Can you work these out from the model? Positions are in its coordinate system, mm. A direction names the side the tool comes from. Coordinates: 2 decimals unless noted, no trailing zeros. Loops run counter-clockwise (first coordinate to the right, second up) from the corner with the lowest first, then second, coordinate; pieces in that order, holes last. Notation, with made-up numbers: (40, -28.5) -> (77, -28.5) arc R23 ccw to (77, 9.5) -> close; hole circle Ø6 at (-19, 16.25). An arc over 180 degrees is marked (long way). Put each result on its own line as item: value. Start each with the question number.
Item 1: If we section it at C-C on z = 133: Please give me the cut outline in (x, y) (3 decimals), plus the area to 3 significant figures.
Item 2: For faces 5 (the flat face through (133, 36, -152.4)), 6 (the flat face through (114.3, 36, 134)), 7 (the flat face through (133, 36, 114.3)), 8 (the flat face through (134, 0, 134)), 9 (the flat face through (-114.3, 104, -134)), which set-ups out of +Z, -Z, +X, -X, +Y, -Y let a thin tool reach every point of the face, with its end or its side?
Item 3: We'd pull the mould along Z, two halves only. Please class faces 1 (the flat face through (-133, 36, 152.4)), 2 (the flat face through (2, 105, -152.4)), 3 (the flat face through (-152.4, 36, 134)), 4 (the flat face through (-152.4, 105, -2)): pulls with the +Z half, pulls with the -Z half, needs draft (parallel to the pull), parting line crosses it, or undercut.
Item 4: Will these pins go through, and if not, where does the flat tip stop? P1, Ø2, axis at x = -43.5, z = 49, coming from the -Y side; P2, Ø12, axis at x = 122.5, z = -44.5, coming from the +Y side; P3, Ø19, axis at y = 21, z = -125.5, coming from the +X side.
Item 5: If we section it at A-A on y = 56.5: Please give me the cut outline in (x, z).
Item 6: If we section it at B-B on y = 100: Please give me the cut outline in (x, z), plus the area to 3 significant figures.
Item 7: If we section it at D-D on x = 137: Please give me the cut outline in (y, z) (3 decimals), plus the area to 3 significant figures.
Item 8: Please list where these lines run through material, in increasing order: L1, parallel to X at y = 87, z = 33; L2, parallel to X at y = 69.5, z = -149.5. Write a range as from..to.
Autodesk Inventor part; units mm, degrees
ref_plane "YZ Plane" through (0, 0, 0) normal (1, 0, 0) x (0, 1, 0)
ref_plane "XZ Plane" through (0, 0, 0) normal (0, 1, 0) x (-1, 0, 0)
ref_plane "XY Plane" through (0, 0, 0) normal (0, 0, 1) x (1, 0, 0)
sketch "Sketch1" plane through (0, 0, 0) normal (0, 1, 0) x (-1, 0, 0)
  line L0 (-152.4, 152.4) -> (152.4, 152.4) construction
  line L1 (152.4, 152.4) -> (152.4, -152.4) construction
  line L2 (152.4, -152.4) -> (-152.4, -152.4) construction
  line L3 (-152.4, -152.4) -> (-152.4, 152.4) construction
  line L4 (-152.4, 152.4) -> (152.4, -152.4) construction
  line L5 (152.4, 152.4) -> (-152.4, -152.4) construction
  line L6 (152.4, -152.4) -> (114.3, -152.4)
  line L7 (114.3, -152.4) -> (114.3, -114.3)
  line L8 (114.3, -114.3) -> (152.4, -114.3)
  line L9 (152.4, -114.3) -> (152.4, -152.4)
  line L10 (152.4, 152.4) -> (152.4, 114.3)
  line L11 (152.4, 114.3) -> (114.3, 114.3)
  line L12 (114.3, 114.3) -> (114.3, 152.4)
  line L13 (114.3, 152.4) -> (152.4, 152.4)
  line L14 (-152.4, 152.4) -> (-114.3, 152.4)
  line L15 (-114.3, 152.4) -> (-114.3, 114.3)
  line L16 (-114.3, 114.3) -> (-152.4, 114.3)
  line L17 (-152.4, 114.3) -> (-152.4, 152.4)
  line L18 (-152.4, -152.4) -> (-152.4, -114.3)
  line L19 (-152.4, -114.3) -> (-114.3, -114.3)
  line L20 (-114.3, -114.3) -> (-114.3, -152.4)
  line L21 (-114.3, -152.4) -> (-152.4, -152.4)
  point P0 (0, 0)
  dimension "d0" = 304.8
  dimension "d1" = 304.8
  dimension "d2" = 38.1
  dimension "d5" = 360
extrude "Extrusion1" add sketch "Sketch1" along normal blind 127
sketch "Sketch2" plane through (0, 127, 0) normal (0, 1, 0) x (1, 0, 0)
  line L0 (-114.3, 152.4) -> (-152.4, 152.4)
  line L1 (-152.4, 152.4) -> (-152.4, 114.3)
  line L2 (-152.4, 114.3) -> (-114.3, 114.3)
  line L3 (-114.3, 114.3) -> (-114.3, 152.4)
  line L4 (152.4, 114.3) -> (152.4, 152.4)
  line L5 (152.4, 152.4) -> (114.3, 152.4)
  line L6 (114.3, 152.4) -> (114.3, 114.3)
  line L7 (114.3, 114.3) -> (152.4, 114.3)
  line L8 (114.3, -152.4) -> (152.4, -152.4)
  line L9 (152.4, -152.4) -> (152.4, -114.3)
  line L10 (152.4, -114.3) -> (114.3, -114.3)
  line L11 (114.3, -114.3) -> (114.3, -152.4)
  line L12 (-152.4, -114.3) -> (-152.4, -152.4)
  line L13 (-152.4, -152.4) -> (-114.3, -152.4)
  line L14 (-114.3, -152.4) -> (-114.3, -114.3)
  line L15 (-114.3, -114.3) -> (-152.4, -114.3)
  line L16 (0, 231.14) -> (0, -231.14)
  line L17 (231.14, 0) -> (-231.14, 0)
  line L18 (-152.4, 152.4) -> (-152.4, -152.4)
  line L19 (-152.4, -152.4) -> (152.4, -152.4)
  line L20 (152.4, -152.4) -> (152.4, 152.4)
  line L21 (152.4, 152.4) -> (-152.4, 152.4)
  line L22 (-165.1, 165.1) -> (-165.1, -165.1)
  line L23 (-165.1, -165.1) -> (165.1, -165.1)
  line L24 (165.1, -165.1) -> (165.1, 165.1)
  line L25 (165.1, 165.1) -> (-165.1, 165.1)
  point P0 (0, 0)
  dimension "d9" = 12.7
extrude "Extrusion2" add sketch "Sketch2" against normal blind 57.15 contours L0 L1 L18 L17 L22 L25 L16 L21 | L16 L25 L24 L17 L20 L4 L5 L21 | L18 L12 L13 L19 L16 L23 L22 L17 | L19 L8 L9 L20 L17 L24 L23 L16
sketch "Sketch3" plane through (0, 69.85, 0) normal (0, -1, 0) x (1, 0, 0)
  line L0 (-165.1, 165.1) -> (165.1, 165.1)
  line L1 (-165.1, -165.1) -> (-165.1, 165.1)
  line L2 (-165.1, 165.1) -> (165.1, 165.1)
  line L3 (165.1, 165.1) -> (165.1, -165.1)
  line L4 (165.1, -165.1) -> (-165.1, -165.1)
  line L5 (114.3, 152.4) -> (-114.3, 152.4)
  line L6 (-114.3, 152.4) -> (-114.3, 114.3)
  line L7 (-114.3, 114.3) -> (-152.4, 114.3)
  line L8 (-152.4, 114.3) -> (-152.4, -114.3)
  line L9 (-152.4, -114.3) -> (-114.3, -114.3)
  line L10 (-114.3, -114.3) -> (-114.3, -152.4)
  line L11 (-114.3, -152.4) -> (114.3, -152.4)
  line L12 (114.3, -152.4) -> (114.3, -114.3)
  line L13 (114.3, -114.3) -> (152.4, -114.3)
  line L14 (152.4, -114.3) -> (152.4, 114.3)
  line L15 (152.4, 114.3) -> (114.3, 114.3)
  line L16 (114.3, 114.3) -> (114.3, 152.4)
  point P0 (0, 0)
extrude "Extrusion3" add sketch "Sketch3" against normal blind 12.7 contours L16 L15 L14 L13 L12 L11 L10 L9 L8 L7 L6 L5
chamfer "Chamfer1" distance 3.175 angle 45 16 edges at (-152.4, 0, 133.35) (-133.35, 0, 152.4) (-114.3, 0, 133.35) (-133.35, 0, 114.3) (-152.4, 0, -133.35) (-133.35, 0, -114.3) (-114.3, 0, -133.35) (-133.35, 0, -152.4) (114.3, 0, -133.35) (133.35, 0, -152.4) (133.35, 0, -114.3) (152.4, 0, -133.35) (133.35, 0, 114.3) (114.3, 0, 133.35) (133.35, 0, 152.4) (152.4, 0, 133.35)
properties part number "Pen"
Solutions:
1. outline: (-165.1, 69.85) -> (-152.4, 69.85) -> (-152.4, 3.175) -> (-149.225, 0) -> (-117.475, 0) -> (-114.3, 3.175) -> (-114.3, 69.85) -> (114.3, 69.85) -> (114.3, 3.175) -> (117.475, 0) -> (149.225, 0) -> (152.4, 3.175) -> (152.4, 69.85) -> (165.1, 69.85) -> (165.1, 127) -> (114.3, 127) -> (114.3, 82.55) -> (-114.3, 82.55) -> (-114.3, 127) -> (-165.1, 127) -> close
1. area: 14,000 mm^2
2. face 5: -Z, +X, -X, -Y
2. face 6: +Z, -Z, -Y
2. face 7: +X, -X, -Y
2. face 8: +Z, -Z, +X, -X, -Y
2. face 9: +Y
3. face 1: pulls with the +Z half
3. face 2: undercut
3. face 3: needs draft
3. face 4: undercut
4. P1: y = 69.85
4. P2: y = 82.55
4. P3: x = 152.4
5. outline: (-152.4, -152.4) -> (-114.3, -152.4) -> (-114.3, -114.3) -> (-152.4, -114.3) -> close; (-152.4, 114.3) -> (-114.3, 114.3) -> (-114.3, 152.4) -> (-152.4, 152.4) -> close; (114.3, -152.4) -> (152.4, -152.4) -> (152.4, -114.3) -> (114.3, -114.3) -> close; (114.3, 114.3) -> (152.4, 114.3) -> (152.4, 152.4) -> (114.3, 152.4) -> close
6. outline: (-165.1, -165.1) -> (165.1, -165.1) -> (165.1, 165.1) -> (-165.1, 165.1) -> close; hole (-152.4, -114.3) -> (-114.3, -114.3) -> (-114.3, -152.4) -> (114.3, -152.4) -> (114.3, -114.3) -> (152.4, -114.3) -> (152.4, 114.3) -> (114.3, 114.3) -> (114.3, 152.4) -> (-114.3, 152.4) -> (-114.3, 114.3) -> (-152.4, 114.3) -> close
6. area: 21,900 mm^2
7. outline: (0, -149.225) -> (3.175, -152.4) -> (69.85, -152.4) -> (69.85, -165.1) -> (127, -165.1) -> (127, -114.3) -> (82.55, -114.3) -> (82.55, 114.3) -> (127, 114.3) -> (127, 165.1) -> (69.85, 165.1) -> (69.85, 152.4) -> (3.175, 152.4) -> (0, 149.225) -> (0, 117.475) -> (3.175, 114.3) -> (69.85, 114.3) -> (69.85, -114.3) -> (3.175, -114.3) -> (0, -117.475) -> close
7. area: 14,000 mm^2
8. L1: -165.1..-152.4, 152.4..165.1
8. L2: -152.4..-114.3, 114.3..152.4
